```python
from build123d import *

# Parameters (mm, degrees)
DODANIE_WYCI_GNI_CIE1_DEPTH = 2
SZKIC8_R                    = 5
SZKIC8_R_2                  = 4
EXTRUDE_THIN1_DEPTH         = 10
SKETCH1_R                   = 2.5
CUT_EXTRUDE1_DEPTH          = 20


with BuildPart() as part:
    # Szkic7 → Dodanie-wyci_gni_cie1 (new body)
    with BuildSketch(Plane(origin=(0, 0, 617.999346089), x_dir=(-1, 0, 0), z_dir=(0, 0, -1))):
        with BuildLine():
            Line((-1236.2588409, -248.22109889), (-1242.917839996, -226.217062929))
            ThreePointArc((-1242.917839996, -226.217062929), (-1236.243055057, -213.749214437), (-1223.775206565, -220.423999377))
            Line((-1223.775206565, -220.423999377), (-1216.726590952, -243.715486458))
            add(Edge.make_bspline(
                [(-1216.726590952, -243.715486458), (-1223.443292113, -241.147709702), (-1231.151179112, -242.879902365), (-1236.2588409, -248.22109889)],
                knots=[0.154038794, 0.154038794, 0.154038794, 0.154038794, 0.334986093, 0.334986093, 0.334986093, 0.334986093], degree=3, weights=[0.573668424, 0.481060845, 0.475765067, 0.557781088]))
        make_face()
    extrude(amount=DODANIE_WYCI_GNI_CIE1_DEPTH)

    # Szkic8 → Extrude-Thin1 (add)
    with BuildSketch(Plane(origin=(0, 0, 615.999346089), x_dir=(-1, 0, 0), z_dir=(0, 0, -1))):
        with Locations((-1233.504191335, -222.034079566)):
            Circle(SZKIC8_R)
        with Locations((-1233.504191335, -222.034079566)):
            Circle(SZKIC8_R_2, mode=Mode.SUBTRACT)
    extrude(amount=EXTRUDE_THIN1_DEPTH)

    # Sketch1 → Cut-Extrude1 (cut)
    with BuildSketch(Plane(origin=(43.382097596, 143.352059634, 0), x_dir=(0.957131672, -0.289653178, 0), z_dir=(0.289653178, 0.957131672, 0))):
        with Locations((1244.938805213, -609.999346089)):
            Circle(SKETCH1_R)
    extrude(amount=-CUT_EXTRUDE1_DEPTH, mode=Mode.SUBTRACT)


solid = part.part
```
Geometry check sheet. Reference: the model listing, model coordinates, mm. A direction names the side the tool comes from. Round coordinates to 2 decimals unless told otherwise and drop trailing zeros. Loops run counter-clockwise (first coordinate to the right, second up) from the corner with the lowest first, then second, coordinate; pieces in that order, holes last. Notation, with made-up numbers: (50.5, 47) -> (104.5, 47) arc R19 ccw to (104.5, 74) -> close; hole circle Ø4 at (24, -2.75). An arc over 180 degrees is marked (long way). Use a Markdown table: item, result.
(1) Sectioned sample at A-A (z = 612). Enter the section's corners in (x, y), then the cut area to 3 significant figures.
Calculated:
| item | result |
|---|---|
| outline | (1230.69, -226.17) -> (1231, -225.15) arc R4 cw to (1233.14, -218.05) -> (1233.45, -217.03) arc R5 ccw to start; (1233.56, -227.03) arc R5 ccw to (1236.32, -217.9) -> (1236.01, -218.92) arc R4 cw to (1233.86, -226.02) -> close |
| area | 22.2 mm² |
(2) Go/stop test with flat-tipped pins: P1, Ø2, axis at y = -241.5, z = 613, coming from the -X side; P2, Ø1, axis at y = -223, z = 614, coming from the -X side; P3, Ø4, axis at x = 1232.5, y = -221, coming from the -Z side. Record where each tip stops, or that it passes through.
Calculated:
| item | result |
|---|---|
| P1 | through |
| P2 | x = 1228.53 |
| P3 | z = 616 |
(3) Sectioned sample at D-D (x = 1239.25). Enter the section's corners in (y, z), then the cut area to 3 significant figures.
Calculated:
| item | result |
|---|---|
| outline | (-238.34, 616) -> (-215.25, 616) -> (-215.25, 618) -> (-238.34, 618) -> close |
| area | 46.2 mm² |
(4) Set-up check for faces 1 (the flat face through (1233, -222, 615.999)), 2 (the flat face through (1230, -231, 617.999)): record each of +Z, -Z, +X, -X, +Y, -Y from which the full face is reachable in a straight line by a thin tool's end or side.
Calculated:
| item | result |
|---|---|
| face 1 | -Z |
| face 2 | +Z, +X, -X, +Y, -Y |
(5) Mould release check, pull along Y, two halves, no side actions. Record for faces 3 (the cylindrical face through (1238.5, -221.8, 611.1)), 4 (the cylindrical face through (1230.568, -225.375, 608.31)), 5 (the flat face through (1230, -231, 615.999)): released by +Y, released by -Y, zero draft, split by the parting line, or undercut.
Calculated:
| item | result |
|---|---|
| face 3 | split by the parting line |
| face 4 | undercut |
| face 5 | zero draft |
(6) Sectioned sample at C-C (y = -223). Enter the section's corners in (x, z), then the cut area to 3 significant figures.
Calculated:
| item | result |
|---|---|
| outline | (1223, 616) -> (1228.6, 616) -> (1228.6, 606) -> (1229.62, 606) -> (1229.62, 616) -> (1237.39, 616) -> (1237.39, 606) -> (1238.41, 606) -> (1238.41, 616) -> (1243.34, 616) -> (1243.34, 618) -> (1223, 618) -> close |
| area | 61.2 mm² |
(7) Sectioned sample at B-B (z = 608). Enter the section's corners in (x, y).
Calculated:
| item | result |
|---|---|
| outline | (1230.69, -226.16) -> (1230.99, -225.15) arc R4 cw to (1233.14, -218.05) -> (1233.45, -217.03) arc R5 ccw to start; (1233.56, -227.03) arc R5 ccw to (1236.32, -217.9) -> (1236.01, -218.92) arc R4 cw to (1233.87, -226.02) -> close |
(8) Scan lines: probe 1 along Z at (x, y) = (1238.5, -229.5); probe 2 along X at (y, z) = (-224.5, 611.25); probe 3 along X at (y, z) = (-221, 615.25). Record each from-to range of solid material in increasing order.
Calculated:
| item | result |
|---|---|
| probe 1 | 616 to 618 |
| probe 2 | 1229.15 to 1230.35, 1236.65 to 1237.85 |
| probe 3 | 1228.61 to 1229.64, 1237.37 to 1238.4 |
